Could you check a few things on this model? Use its own coordinates, in mm. Face numbers are marked on the shaded views. A direction names the side the tool comes from. Coordinates: 2 decimals unless noted, no trailing zeros. Loops run counter-clockwise (first coordinate to the right, second up) from the corner with the lowest first, then second, coordinate; pieces in that order, holes last. Notation, with made-up numbers: (-35.75, 20) -> (10.25, 20) arc R21 ccw to (10.25, 26) -> close; hole circle Ø1 at (45, -38). An arc over 180 degrees is marked (long way). One line per question, with ' | ' between items. Start each with the question number.
(1) If I drill on line 1 along Y through (x, z) = (0, -34) (1 decimal); line 2 along Z through (x, y) = (-7, 11); line 3 along X through (y, z) = (-3, 32.5), over which ranges is the centre line in solid material (lowest first)?
(2) Suppose I cut it at C-C (y = -16). Please give me the cut outline in (x, z).
(3) Which directions (+Z, -Z, +X, -X, +Y, -Y) give clear straight access to the entire face, cutting with the end or side of a thin tool? Please do the marked faces 4 and 5.
(4) If we mould it in two halves opening along Z, with no side actions, what happens to the marked faces 1, 2 and 3? For each: pulls with the +Z half, pulls with the -Z half, needs draft (parallel to the pull), parting line crosses it, or undercut.
(5) Suppose I cut it at A-A (x = 0). Give the number of separate pieces and of enclosed holes in the cut face, plus the area to 3 significant figures.
(6) Suppose I cut it at B-B (x = 13). Please give me the cut outline in (y, z).
(7) I'm going to push flat-ended pins straight in: pin 1 Ø1.5 at (y, z) = (8, -25) entering from -X; pin 2 Ø1.5 at (x, z) = (-1.5, -22.5) entering from -Y; pin 3 Ø2 at (x, y) = (29, -25) entering from +Z (1 decimal); pin 4 Ø3 at (x, z) = (19, 31) entering from +Y. Where does each tip first touch, or does it pass through?
```python
from build123d import *

# Parameters (mm, degrees)
BOSS_EXTRUDE1_DEPTH     = 38.1
FILLET1_R               = 3.175
FILLET2_R               = 6.35
FILLET3_R               = 6.35
FILLET4_R               = 3.175
CUT_EXTRUDE2_DEPTH      = 97.278232488
CUT_EXTRUDE2_DEPTH_BACK = 97.278232488
SKETCH4_R               = 9.525
CUT_EXTRUDE4_DEPTH      = 19.05
FILLET5_R               = 3.175


with BuildPart() as part:
    # Sketch1 → Boss-Extrude1 (new, symmetric)
    with BuildSketch(Plane.XY):
        with BuildLine():
            Line((14.2875, 0), (20.6375, 0))
            ThreePointArc((20.6375, 0), (25.87049136, -24.319115263), (34.567577214, -47.625))
            Line((34.567577214, -47.625), (29.343435198, -47.625))
            ThreePointArc((29.343435198, -47.625), (22.762716722, -30.40866876), (18.016295413, -12.599137554))
            ThreePointArc((18.016295413, -12.599137554), (14.73137517, -9.023483479), (10.017434273, -10.187426899))
            ThreePointArc((10.017434273, -10.187426899), (-13.17681199, 5.523068172), (14.2875, 0))
        make_face()
    extrude(amount=BOSS_EXTRUDE1_DEPTH, both=True)

    # Fillet1
    fillet1_edges = [part.edges().sort_by_distance(p)[0] for p in [
        (14.2875, 0, 0),
    ]]
    fillet(fillet1_edges, radius=FILLET1_R)

    # Fillet2
    fillet2_edges = [part.edges().sort_by_distance(p)[0] for p in [
        (31.955506206, -47.625, 38.1),
    ]]
    fillet(fillet2_edges, radius=FILLET2_R)

    # Fillet3
    fillet3_edges = [part.edges().sort_by_distance(p)[0] for p in [
        (31.955506206, -47.625, -38.1),
    ]]
    fillet(fillet3_edges, radius=FILLET3_R)

    # Fillet4
    # the kernel refuses this fillet: 3.175 mm, written as the material it takes off along each edge
    with BuildSketch(Plane(origin=(29.343435198, -47.625, -36.993879976), x_dir=(-0.3999574931440754, 0.9165336893305706, 0), z_dir=(0, 0, 1))) as fillet4_piece_1:
        with BuildLine():
            CenterArc((2.078655126, -3.174943765), FILLET4_R, 89.658986775, 66.765492029)
            Line((-0.831339338, -1.905078724), (0, 0))
            ThreePointArc((0, 0), (1.048775995, 0.003121064), (2.09755199, 0))
        make_face()
    extrude(amount=73.987759951, mode=Mode.SUBTRACT)

    # Sketch4 → Cut-Extrude2 (cut, two sides: drawn at the far end of the back side and taken through both)
    with BuildSketch(Plane.XY.offset(38.1).offset(-CUT_EXTRUDE2_DEPTH_BACK)):
        Circle(SKETCH4_R)
    extrude(amount=CUT_EXTRUDE2_DEPTH + CUT_EXTRUDE2_DEPTH_BACK, mode=Mode.SUBTRACT)

    # Sketch6 → Cut-Extrude4 (cut, symmetric)
    with BuildSketch(Plane.XY):
        with BuildLine():
            Line((29.343435198, -47.625), (31.081601096, -47.625))
            ThreePointArc((31.081601096, -47.625), (22.620737822, -24.512971667), (17.493272193, -0.440972222))
            Line((17.493272193, -0.440972222), (20.6375, 0))
            Line((20.6375, 0), (17.171437949, 0))
            ThreePointArc((17.171437949, 0), (15.140701126, 0.734358086), (14.049358322, 2.597727273))
            ThreePointArc((14.049358322, 2.597727273), (-13.625992377, 4.297090643), (10.017434273, -10.187426899))
            ThreePointArc((10.017434273, -10.187426899), (14.73137517, -9.023483479), (18.016295413, -12.599137554))
            ThreePointArc((18.016295413, -12.599137554), (22.762716722, -30.40866876), (29.343435198, -47.625))
        make_face()
    extrude(amount=CUT_EXTRUDE4_DEPTH, both=True, mode=Mode.SUBTRACT)

    # Fillet5
    # the kernel refuses this fillet: 3.175 mm, written as the material it takes off along each edge
    with BuildSketch(Plane(origin=(17.493272193, -0.440972222, -19.05), x_dir=(0.14805284588297285, -0.9889794511646602, 0), z_dir=(0, 0, 1))) as fillet5_piece_1:
        with BuildLine():
            CenterArc((3.204535532, 3.174863883), FILLET5_R, 179.469453196, 91.061093608)
            Line((0.029671649, 3.204263291), (0, 0))
            ThreePointArc((0, 0), (1.61696747, -0.007486442), (3.23393494, 0))
        make_face()
    extrude(amount=38.1, mode=Mode.SUBTRACT)


solid = part.part
```
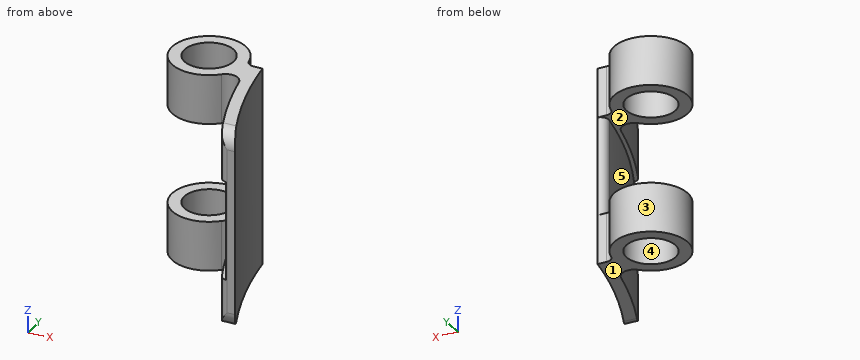
Checks:
1) line 1: y = -14.3 to -9.5, 9.5 to 14.3 | line 2: z = -38.1 to -19.05, 19.05 to 38.1 | line 3: x = -13.97 to -9.04, 9.04 to 21.09
2) outline: (18.77, -38.1) -> (23.66, -38.1) -> (23.66, 38.1) -> (18.77, 38.1) -> (18.77, 19.05) -> (20.4, 19.05) -> (20.4, -19.05) -> (18.77, -19.05) -> close
3) face 4: +Z, -Z | face 5: -X, -Y
4) face 1: pulls with the -Z half | face 2: undercut | face 3: needs draft
5) separate pieces: 4 | enclosed holes: 0 | area: 363 mm^2
6) outline: (-8.83, -38.1) -> (5.93, -38.1) -> (5.93, -19.05) -> (-8.83, -19.05) -> close; (-8.83, 19.05) -> (5.93, 19.05) -> (5.93, 38.1) -> (-8.83, 38.1) -> close
7) pin 1: stops at x = -12.31 | pin 2: stops at y = -14.27 | pin 3: passes through | pin 4: stops at y = 0
